```python
from build123d import *

# Parameters (mm, degrees)
SKETCH1_R            = 4.85
BASE_DEPTH           = 7.4
TOOTHCUT_DEPTH       = 11.089846381
TEETHCUTS_COUNT      = 16
SKETCH3_W            = 6.5
SKETCH3_H            = 5.1
SHAFTHOLE_DEPTH      = 16.516120649
SHAFTHOLE_DEPTH_BACK = 16.516120649
SKETCH4_R            = 2.5


with BuildPart() as part:
    # Sketch1 → Base (new body)
    with BuildSketch(Plane.XY):
        Circle(SKETCH1_R)
    extrude(amount=BASE_DEPTH)

    # Sketch2 → ToothCut (cut, through all)
    with BuildSketch(Plane.XY.offset(7.4)):
        with BuildLine():
            Line((-0.758707155, 4.790288452), (-0.789765541, 5.545021864))
            Line((-0.789765541, 5.545021864), (0.920739556, 5.545021864))
            Line((0.920739556, 5.545021864), (0.758707155, 4.790288452))
            ThreePointArc((0.758707155, 4.790288452), (0.754679502, 4.790924634), (0.750651316, 4.79155743))
            ThreePointArc((0.750651316, 4.79155743), (0.639888447, 4.765166202), (0.579571668, 4.668590862))
            ThreePointArc((0.579571668, 4.668590862), (0.550654119, 4.546148399), (0.506591342, 4.428305906))
            ThreePointArc((0.506591342, 4.428305906), (0, 4.1), (-0.506591342, 4.428305906))
            ThreePointArc((-0.506591342, 4.428305906), (-0.550654119, 4.546148399), (-0.579571668, 4.668590862))
            ThreePointArc((-0.579571668, 4.668590862), (-0.639888447, 4.765166202), (-0.750651316, 4.79155743))
            ThreePointArc((-0.750651316, 4.79155743), (-0.754679502, 4.790924634), (-0.758707155, 4.790288452))
        make_face()
    toothcut = extrude(amount=-TOOTHCUT_DEPTH, mode=Mode.SUBTRACT)

    # TeethCuts: ToothCut ×16 about axis
    teethcuts_axis = Axis((0, 0, 0), (0, 0, 1))
    for i in range(1, TEETHCUTS_COUNT):
        add(toothcut.rotate(teethcuts_axis, i * 360 / TEETHCUTS_COUNT), mode=Mode.SUBTRACT)

    # Sketch3 → Body (revolve)
    with BuildSketch(Plane(origin=(0, 0, 0), x_dir=(1, 0, 0), z_dir=(0, 1, 0)), mode=Mode.PRIVATE) as body_sk:
        Polygon((0, 0), (0, 1.5), (-6.5, 1.5), (-6.5, 0.5), (-5.5, 0), align=None)
        with Locations((-3.25, -9.95)):
            Rectangle(SKETCH3_W, SKETCH3_H)
    revolve(body_sk.sketch.rotate(Axis((0, 0, 12.5), (0, 0, -1)), 180), axis=Axis((0, 0, 12.5), (0, 0, -1)))

    # Sketch4 → ShaftHole (cut, two sides: drawn at the far end of the back side and taken through both)
    with BuildSketch(Plane.XY.offset(-SHAFTHOLE_DEPTH_BACK)):
        Circle(SKETCH4_R)
    extrude(amount=SHAFTHOLE_DEPTH + SHAFTHOLE_DEPTH_BACK, mode=Mode.SUBTRACT)


solid = part.part
```
Here's how the part is built. I have some questions about the finished solid (model axes, mm). A direction names the side the tool comes from. Round coordinates to 2 decimals unless told otherwise and drop trailing zeros. Write each loop counter-clockwise with the first axis right and the second up, starting at its lowest first coordinate (ties: lowest second). Pieces come first, ordered by that corner, then holes.
Q1. If we mould it in two halves opening along Y, with no side actions, what happens to faces 1 (the cylindrical face through (-5.158, 3.955, 9.914)), 2 (the cylindrical face through (3.79, 1.56, 3.75)), 3 (the cylindrical face through (0, -4.1, 3.8)), 4 (the cylindrical face through (-0.54, -2.44, 5.4))? For each: +Y half, -Y half, draft (parallel to the pull), parting line (faces both ways), or undercut.
Q2. If we section it at A-A on y = 0: Write out the boundary of the cut face in (x, z).
Q3. Will these pins go through, and if not, where does the flat tip stop? P1, Ø4, axis at y = 3.5, z = 10.5, coming from the +X side; P2, Ø2, axis at y = 1.5, z = 2.5, coming from the +X side; P3, Ø1, axis at x = -1, y = -0.5, coming from the +Z side.
Q4. Which directions (+Z, -Z, +X, -X, +Y, -Y) give clear straight access to the entire face, cutting with the end or side of a thin tool? Please do faces 5 (the flat face through (1.4, 4.2, 7.4)), 6 (the cylindrical face through (4.1, 0, 3.8)), 7 (the cylindrical face through (0, 4.1, 3.8)), 8 (the cylindrical face through (-4.1, 0, 3.8)).
Q5. Please list where these lines run through material, in increasing order: probe 1 along Z at (x, y) = (4.5, 2); probe 2 along Y at (x, z) = (0, 4.5).
Q6. If we section it at C-C on z = 8.5: Write out the boundary of the cut face in (x, y).
Answer below:
1. face 1: parting line
1. face 2: undercut
1. face 3: -Y half
1. face 4: undercut
2. outline: (-6.5, -1.5) - (-2.5, -1.5) - (-2.5, 12.5) - (-6.5, 12.5) - (-6.5, 7.4) - (-4.1, 7.4) - (-4.1, 0) - (-5.5, 0) - (-6.5, -0.5) - close; (2.5, -1.5) - (6.5, -1.5) - (6.5, -0.5) - (5.5, 0) - (4.1, 0) - (4.1, 7.4) - (6.5, 7.4) - (6.5, 12.5) - (2.5, 12.5) - close
3. P1: stops at x = 6.32
3. P2: stops at x = 4.79
3. P3: passes through
4. face 5: none
4. face 6: +X
4. face 7: +Y
4. face 8: -X
5. probe 1: z = -1.5 to 0, 7.4 to 12.5
5. probe 2: y = -4.1 to -2.5, 2.5 to 4.1
6. outline: circle Ø13 at (0, 0); hole circle Ø5 at (0, 0)
